Here's how the part is built. I have some questions about the finished solid (model axes, mm). A direction names the side the tool comes from. Coordinates: 2 decimals unless noted, no trailing zeros. Write each loop counter-clockwise with the first axis right and the second up, starting at its lowest first coordinate (ties: lowest second). Pieces come first, ordered by that corner, then holes. Notation, with made-up numbers: (76.5, 29) - (110.5, 29) arc R18 ccw to (110.5, 51) - close; hole circle Ø6 at (87, 18). An arc over 180 degrees is marked (long way). Answer in a Markdown table with one row per item. Add a question column.
Item 1: If I drill on probe 1 along X at (y, z) = (-11, -0.25); probe 2 along X at (y, z) = (5, -0.3); probe 3 along Y at (x, z) = (11, -0.15), over which ranges is the centre line in solid material (lowest first)? Write a range as from..to.
Item 2: I'm going to push a flat-ended pin straight in: pin 1 (5.5 mm diameter, centred on x = -3, y = -17, fed in from -Z). Where does the tip first touch, or does it pass through?
Item 3: Which directions (+Z, -Z, +X, -X, +Y, -Y) give clear straight access to the entire face, cutting with the end or side of a thin tool? Please do faces 5 (the face through (18, 0, 0)), 6 (the face through (24.7, 6.44, 0.24)).
Item 4: We'd pull the mould along X, two halves only. Please class faces 1 (the face through (18, -18, 0)), 2 (the face through (8, -9, -0.5)), 3 (the face through (27.55, -9, 0)), 4 (the face through (22.276, -26.129, -0.246)): +X half, -X half, draft (parallel to the pull), parting line (faces both ways), or undercut.
Item 5: Imagine slicing it at A-A (z = 0.3). Please give me the cut outline in (x, y), plus the area to 3 significant figures.
Item 6: Imagine slicing it at B-B (y = 6). Please give me the cut outline in (x, z), plus the area to 3 significant figures.
Item 7: Imagine slicing it at C-C (x = 1). Please give me the cut outline in (y, z).
from build123d import *

# Parameters (mm, degrees)
SKETCH_1_W      = 37
SKETCH_1_H      = 37
EXTRUDE_1_DEPTH = 1
SKETCH_1_6_W    = 37
SKETCH_1_6_H    = 37
SKETCH_1_6_R    = 9.05
SKETCH_1_6_R_2  = 9
EXTRUDE_3_DEPTH = 0.5
FILLET_1_R      = 10


with BuildPart() as part:
    # Эскиз1 → Бобышка-Вытянуть1 (new body)
    with BuildSketch(Plane.XY):
        with Locations((9.05, -9.05)):
            Rectangle(SKETCH_1_W, SKETCH_1_H)
    extrude(amount=EXTRUDE_1_DEPTH)

    # Эскиз1<6> → Бобышка-Вытянуть3 (add)
    with BuildSketch(Plane.XY):
        with Locations((9.05, -9.05)):
            Rectangle(SKETCH_1_6_W, SKETCH_1_6_H)
        with Locations((18.1, -18.1)):
            Circle(SKETCH_1_6_R, mode=Mode.SUBTRACT)
        Circle(SKETCH_1_6_R_2, mode=Mode.SUBTRACT)
        with Locations((18.1, 0)):
            Circle(SKETCH_1_6_R_2, mode=Mode.SUBTRACT)
        with Locations((0, -18.1)):
            Circle(SKETCH_1_6_R_2, mode=Mode.SUBTRACT)
    extrude(amount=-EXTRUDE_3_DEPTH)

    # Скругление1
    fillet_1_edges = [part.edges().sort_by_distance(p)[0] for p in [
        (-9.45, -27.55, 0.25),
        (-9.45, 9.45, 0.25),
        (27.55, 9.45, 0.25),
        (27.55, -27.55, 0.25),
    ]]
    fillet(fillet_1_edges, radius=FILLET_1_R)


solid = part.part
Here are the results:
| question | item | result |
|---|---|---|
| 1 | probe 1 | x = -9.45..-5.53, 5.53..12.49, 23.71..27.55 |
| 1 | probe 2 | x = -7.77..-7.48, 7.48..10.62, 25.58..25.87 |
| 1 | probe 3 | y = -27.55..-23.71, -12.49..-5.53, 5.53..9.45 |
| 2 | pin 1 | stops at z = 0 |
| 3 | face 5 | -Z |
| 3 | face 6 | +Z, -Z, +X, +Y |
| 4 | face 1 | undercut |
| 4 | face 2 | draft |
| 4 | face 3 | +X half |
| 4 | face 4 | undercut |
| 5 | outline | (-9.45, -17.55) arc R10 ccw to (0.55, -27.55) - (17.55, -27.55) arc R10 ccw to (27.55, -17.55) - (27.55, -0.55) arc R10 ccw to (17.55, 9.45) - (0.55, 9.45) arc R10 ccw to (-9.45, -0.55) - close |
| 5 | area | 1,280 mm2 |
| 6 | outline | (-7.01, -0.5) - (-6.71, -0.5) - (-6.71, 0) - (6.71, 0) - (6.71, -0.5) - (11.39, -0.5) - (11.39, 0) - (24.81, 0) - (24.81, -0.5) - (25.11, -0.5) - (25.11, 1) - (-7.01, 1) - close |
| 6 | area | 34.8 mm2 |
| 7 | outline | (-27.55, -0.5) - (-27.04, -0.5) - (-27.04, 0) - (-9.16, 0) - (-9.16, -0.5) - (-8.94, -0.5) - (-8.94, 0) - (8.94, 0) - (8.94, -0.5) - (9.45, -0.5) - (9.45, 1) - (-27.55, 1) - close |
